The drawing under review shows one solid part. Ordinate dimensions are in mm from its lowest x, y, z. Give positions to 0.01 mm unless a question says otherwise; leave off trailing zeros. Write each loop counter-clockwise with the first axis right and the second up, starting at its lowest first coordinate (ties: lowest second). Pieces come first, ordered by that corner, then holes. Notation, with made-up numbers: M 52.25,43.5 L 104.25,43.5 A13 ccw 104.25,53.5 Z; hole C 54.5,-39.75 d11. An arc over 180 degrees is marked long. One line per item, written item: value. Start each with the question number.
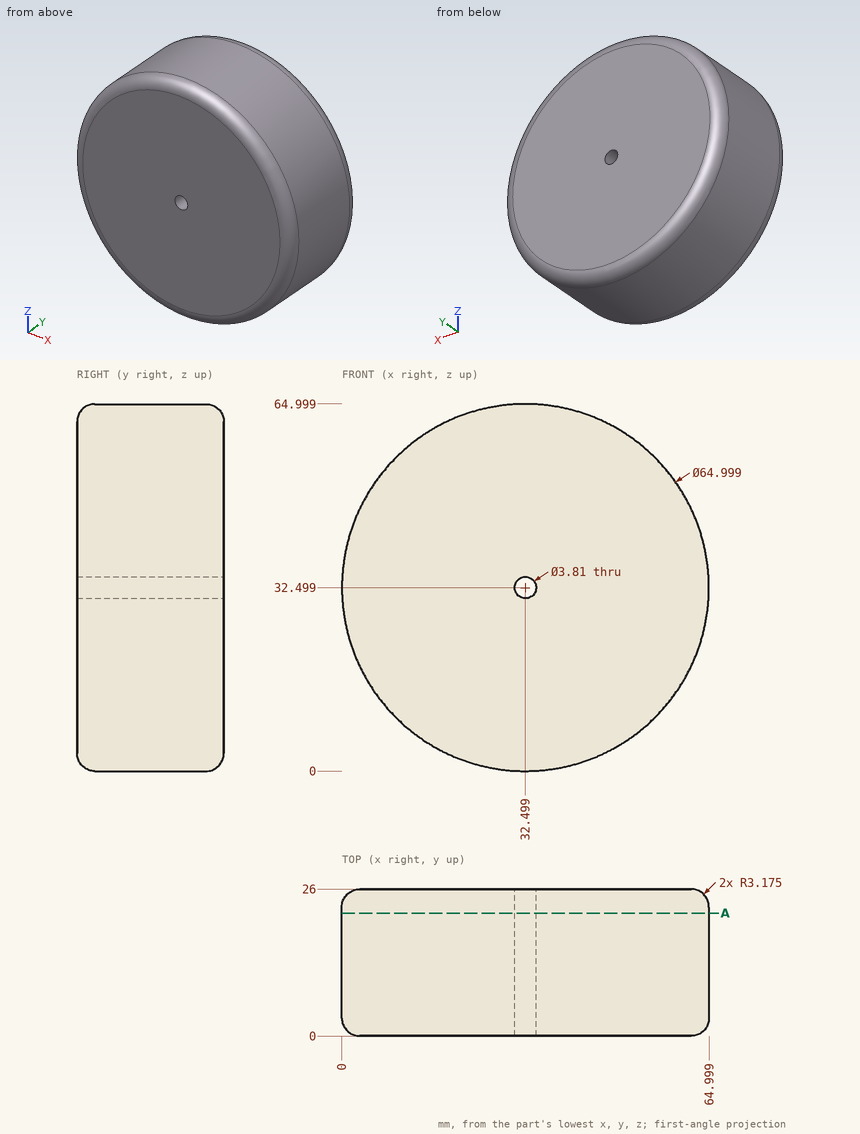
Q1. Wall thickness on line 1 (Z direction, x = 33, y = 24.5); line 2 (X direction, y = 16.75, z = 52.5) (1 decimal); line 3 (X direction, y = 6.5, z = 24): over which ranges is each line inside the solid? List them lowest first. Write a range as from..to.
Q2. Take a section at A-A, the plane y = 21.75. Give the boundary of the cut face in (x, z) (1 decimal), then the cut area to 3 significant figures.
Q3. For P1, Ø12, axis at x = 57.5, y = 18, coming from the -Z side; P2, Ø5, axis at y = 21.5, z = 12, coming from the -X side; P3, Ø8, axis at y = 3.5, z = 25, coming from the -X side, all flat-tipped, find the tip position at first contact; note any pin that passes through.
Results list:
1. line 1: z = 0.48..30.66, 34.34..64.52
1. line 2: x = 6.9..58.1
1. line 3: x = 1.13..63.87
2. outline: C 32.5,32.5 d65; hole C 32.5,32.5 d3.8
2. area: 3,310 mm^2
3. P1: stops at z = 6.13
3. P2: stops at x = 5.44
3. P3: stops at x = 0.19
